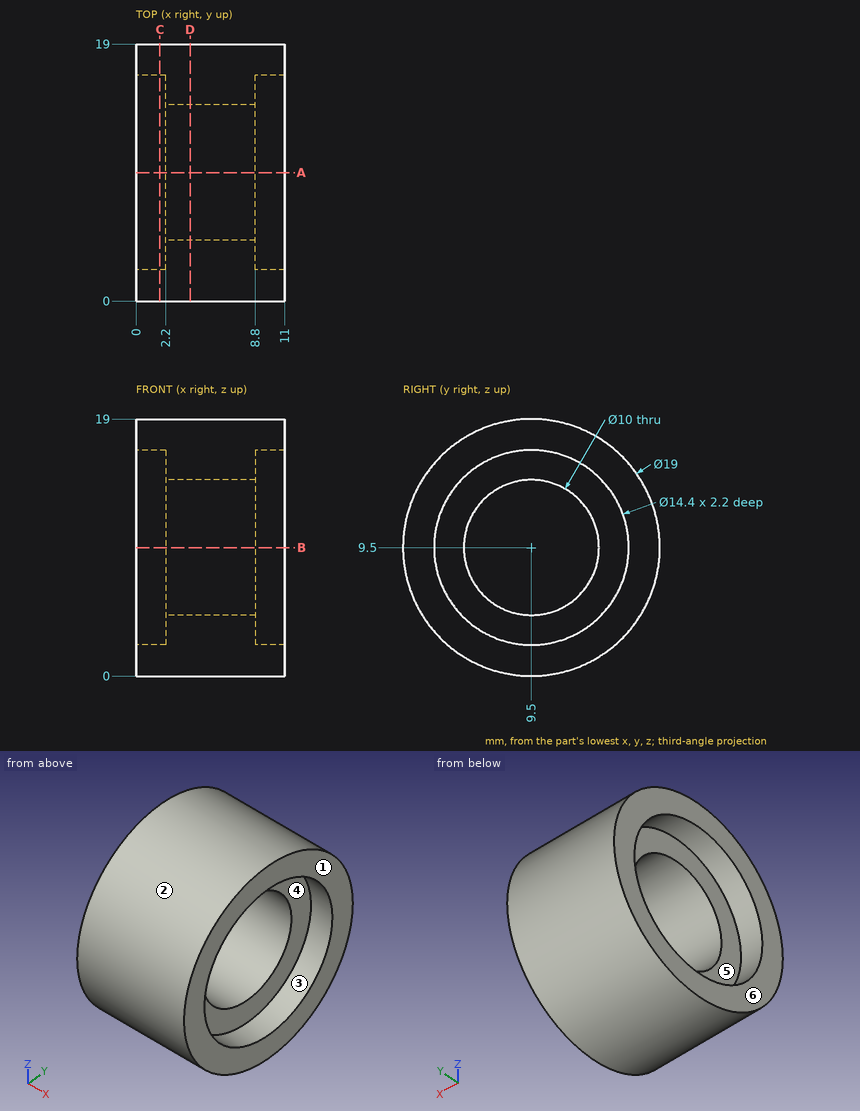
Geometry: see drawing. Coordinates: mm, zero at the bounding-box minimum. A direction names the side the tool comes from. Give positions to 0.01 mm unless a question says otherwise; leave off trailing zeros. Write each loop counter-clockwise with the first axis right and the second up, starting at its lowest first coordinate (ties: lowest second). Pieces come first, ordered by that corner, then holes. Notation, with made-up numbers: M 22,-18 L 60,-18 A25 ccw 60,4 Z; hole C -2.5,-5 d8. An arc over 180 degrees is marked long. Answer in a Markdown table with one row per item. Add a question column.
(1) Section A-A on y = 9.5. Return loops of the section in (x, z), and give its area (3 significant figures).
(2) Mould query, pull axis Z, two halves, no side actions, for the marked faces 1, 2 and 3. Classes: +Z half, -Z half, draft (parallel to the pull), parting line (faces both ways), or undercut.
(3) Reachability of the marked faces 4, 5 and 6 from +Z, -Z, +X, -X, +Y, -Y: full face, straight path, thin tool, end or side. Return the list, or none.
(4) First-contact query: pin 1 (6 mm diameter, centred on x = 2, z = 5, fed in from +Y); pin 2 (9 mm diameter, centred on y = 9.5, z = 9.5, fed in from +X); pin 3 (3 mm diameter, centred on x = 8, y = 2.5, fed in from -Z); pin 4 (7 mm diameter, centred on y = 9.5, z = 6, fed in from -X). Flat tips, straight axial feed; report the tip coordinate or a pass-through.
(5) Section C-C on x = 1.75. Return loops of the section in (y, z), and give its area (3 significant figures).
(6) Ray query, line 1 (Y direction, x = 1.6, z = 9.5); line 2 (Y direction, x = 7.25, z = 9.5); line 3 (X direction, y = 14.5, z = 11). Return the intervals inside material, ascending.
(7) Section D-D on x = 4. Return loops of the section in (y, z).
Result set:
| question | item | result |
|---|---|---|
| 1 | outline | M 0,0 L 11,0 L 11,2.3 L 8.8,2.3 L 8.8,4.5 L 2.2,4.5 L 2.2,2.3 L 0,2.3 Z; M 0,16.7 L 2.2,16.7 L 2.2,14.5 L 8.8,14.5 L 8.8,16.7 L 11,16.7 L 11,19 L 0,19 Z |
| 1 | area | 79.6 mm^2 |
| 2 | face 1 | draft |
| 2 | face 2 | parting line |
| 2 | face 3 | undercut |
| 3 | face 4 | +X |
| 3 | face 5 | -X |
| 3 | face 6 | +Z, -Z, -X, +Y, -Y |
| 4 | pin 1 | stops at y = 18.88 |
| 4 | pin 2 | passes through |
| 4 | pin 3 | stops at z = 1.75 |
| 4 | pin 4 | stops at x = 2.2 |
| 5 | outline | C 9.5,9.5 d19; hole C 9.5,9.5 d14.4 |
| 5 | area | 121 mm^2 |
| 6 | line 1 | y = 0 to 2.3, 16.7 to 19 |
| 6 | line 2 | y = 0 to 4.5, 14.5 to 19 |
| 6 | line 3 | x = 2.2 to 8.8 |
| 7 | outline | C 9.5,9.5 d19; hole C 9.5,9.5 d10 |
